For this review, take the finished solid that the model builds, in its own axes (mm). A direction names the side the tool comes from. Coordinates: 2 decimals unless noted, no trailing zeros. Write each loop counter-clockwise with the first axis right and the second up, starting at its lowest first coordinate (ties: lowest second). Pieces come first, ordered by that corner, then holes.
```python
from build123d import *

# Parameters (mm, degrees)
BOSS_EXTRUDE1_DEPTH = 5
SKETCH3_R           = 1.8
SKETCH3_W           = 20
SKETCH3_H           = 3
SKETCH3_W_2         = 25
SKETCH3_W_3         = 3
SKETCH3_H_2         = 30
ARDUINO_DEPTH       = 6
SKETCH6_R           = 1.8
CUT_EXTRUDE4_DEPTH  = 6
SKETCH8_R           = 1.8
CUT_EXTRUDE5_DEPTH  = 10
SKETCH9_R           = 1.8
SKETCH9_R_2         = 2.5
SKETCH9_W           = 3
SKETCH9_H           = 30
L298N_DEPTH         = 10
SKETCH11_W          = 24
SKETCH11_H          = 5
CUT_EXTRUDE7_DEPTH  = 10
SKETCH12_W          = 100
SKETCH12_H          = 20
CUT_EXTRUDE8_DEPTH  = 10


with BuildPart() as part:
    # Sketch1 → Boss-Extrude1 (new body)
    with BuildSketch(Plane(origin=(0, 0, 0), x_dir=(1, 0, 0), z_dir=(0, 1, 0))):
        with BuildLine():
            Line((100, -40), (100, 10))
            Line((100, 10), (30, 170))
            Line((30, 170), (-30, 170))
            Line((-30, 170), (-100, 10))
            Line((-100, 10), (-100, -40))
            ThreePointArc((-100, -40), (-97.071067812, -47.071067812), (-90, -50))
            Line((-90, -50), (-75, -50))
            Line((-75, -50), (-75, -70))
            Line((-75, -70), (-30, -70))
            Line((-30, -70), (-30, -73))
            Line((-30, -73), (30, -73))
            Line((30, -73), (30, -70))
            Line((30, -70), (75, -70))
            Line((75, -70), (75, -50))
            Line((75, -50), (90, -50))
            ThreePointArc((90, -50), (97.071067812, -47.071067812), (100, -40))
        make_face()
    extrude(amount=BOSS_EXTRUDE1_DEPTH)

    # Sketch3 → arduino (cut, through all)
    with BuildSketch(Plane(origin=(0, 5, 0), x_dir=(1, 0, 0), z_dir=(0, 1, 0))):
        with Locations((-76.120983048, 12.737637313)):
            Circle(SKETCH3_R)
        with Locations((-77.220983048, -35.062362687)):
            Circle(SKETCH3_R)
        with Locations((-25.320983048, -2.462362687)):
            Circle(SKETCH3_R)
        with Locations((-25.320983048, -30.362362687)):
            Circle(SKETCH3_R)
        with Locations((-45.320983048, -41.562362687)):
            Rectangle(SKETCH3_W, SKETCH3_H)
        with Locations((-47.820983048, 19.237637313)):
            Rectangle(SKETCH3_W_2, SKETCH3_H)
        with Locations((-18.820983048, -15.362362687)):
            Rectangle(SKETCH3_W_3, SKETCH3_H_2)
    extrude(amount=-ARDUINO_DEPTH, mode=Mode.SUBTRACT)

    # Sketch6 → Cut-Extrude4 (cut, through all)
    with BuildSketch(Plane(origin=(0, 5, 0), x_dir=(1, 0, 0), z_dir=(0, 1, 0))):
        with Locations((20, 120)):
            Circle(SKETCH6_R)
        with Locations((-20, 120)):
            Circle(SKETCH6_R)
    extrude(amount=-CUT_EXTRUDE4_DEPTH, mode=Mode.SUBTRACT)

    # Sketch8 → Cut-Extrude5 (cut)
    with BuildSketch(Plane(origin=(0, 5, 0), x_dir=(1, 0, 0), z_dir=(0, 1, 0))):
        with Locations((8, 10)):
            Circle(SKETCH8_R)
        with Locations((-8, 10)):
            Circle(SKETCH8_R)
        with Locations((-65, -60)):
            Circle(SKETCH8_R)
        with Locations((65, -60)):
            Circle(SKETCH8_R)
        with Locations((8, -52)):
            Circle(SKETCH8_R)
        with Locations((24, -52)):
            Circle(SKETCH8_R)
        with Locations((40, -52)):
            Circle(SKETCH8_R)
        with Locations((-8, -52)):
            Circle(SKETCH8_R)
        with Locations((-40, -52)):
            Circle(SKETCH8_R)
        with Locations((-24, -52)):
            Circle(SKETCH8_R)
    extrude(amount=-CUT_EXTRUDE5_DEPTH, mode=Mode.SUBTRACT)

    # Sketch9 → l298n (cut)
    with BuildSketch(Plane(origin=(0, 5, 0), x_dir=(1, 0, 0), z_dir=(0, 1, 0))):
        with Locations((20, 72)):
            Circle(SKETCH9_R)
        with Locations((-20, 72)):
            Circle(SKETCH9_R)
        with Locations((51, 10)):
            Circle(SKETCH9_R)
        with Locations((87.998174007, 10.367586933)):
            Circle(SKETCH9_R)
        with Locations((88.36576094, -26.630587074)):
            Circle(SKETCH9_R)
        with Locations((51.367586933, -26.998174007)):
            Circle(SKETCH9_R)
        with Locations((-68.125, 50)):
            Circle(SKETCH9_R)
        with Locations((68.125, 50)):
            Circle(SKETCH9_R)
        with Locations((61, 25)):
            Circle(SKETCH9_R_2)
        with Locations((61.367586933, -41.998174007)):
            Circle(SKETCH9_R_2)
        with Locations((0, 27)):
            Circle(SKETCH9_R_2)
        with Locations((29.5, -10)):
            Rectangle(SKETCH9_W, SKETCH9_H)
    extrude(amount=-L298N_DEPTH, mode=Mode.SUBTRACT)

    # Sketch11 → Cut-Extrude7 (cut)
    with BuildSketch(Plane(origin=(0, 5, 0), x_dir=(1, 0, 0), z_dir=(0, 1, 0))):
        with Locations((-58, -67.5)):
            Rectangle(SKETCH11_W, SKETCH11_H)
        with Locations((58, -67.5)):
            Rectangle(SKETCH11_W, SKETCH11_H)
    extrude(amount=-CUT_EXTRUDE7_DEPTH, mode=Mode.SUBTRACT)

    # Sketch12 → Cut-Extrude8 (cut)
    with BuildSketch(Plane(origin=(0, 5, 0), x_dir=(1, 0, 0), z_dir=(0, 1, 0))):
        with Locations((0, 160)):
            Rectangle(SKETCH12_W, SKETCH12_H)
    extrude(amount=-CUT_EXTRUDE8_DEPTH, mode=Mode.SUBTRACT)


solid = part.part
```
Q1. Add section B-B (z = -78). State the section outline as (x, y) points.
Ans:
outline: (-70.25, 0) - (70.25, 0) - (70.25, 5) - (-70.25, 5) - close
Q2. Add section C-C (y = 2.9). Give the number of separate pieces and of enclosed holes in the cut face, then the cut area to 3 significant figures.
Ans:
separate pieces: 1
enclosed holes: 31
area: 33,700 mm2
Q3. Add section D-D (z = -101). State the section outline as (x, y) points, then the cut area to 3 significant figures.
Ans:
outline: (-60.19, 0) - (60.19, 0) - (60.19, 5) - (-60.19, 5) - close
area: 602 mm2
Q4. For probe 1 along Z at (x, y) = (20, 1.5); probe 2 along Z at (x, y) = (8, 3.65); probe 3 along Z at (x, y) = (65, 2.55), list the stretches that pass through material, from the lowest coordinate up.
Ans:
probe 1: z = -150 to -121.8, -118.2 to -73.8, -70.2 to 73
probe 2: z = -150 to -11.8, -8.2 to 50.2, 53.8 to 73
probe 3: z = -90 to 58.2, 61.8 to 65
Q5. Add section A-A (x = -48.5). State the section outline as (y, z) points, then the cut area to 3 significant figures.
Ans:
outline: (0, -127.71) - (5, -127.71) - (5, -20.74) - (0, -20.74) - close; (0, -17.74) - (5, -17.74) - (5, 40.06) - (0, 40.06) - close; (0, 43.06) - (5, 43.06) - (5, 65) - (0, 65) - close
area: 934 mm2
Q6. Clearance check with flat-ended pins moving along their axes: pin 1 Ø4 at (x, z) = (-77.22, 35.06) entering from -Y; pin 2 Ø2 at (y, z) = (3.5, -12.5) entering from -X; pin 3 Ø1.5 at (y, z) = (2.5, 71.5) entering from +X. State where each tip first meets the part, or that it passes through.
Ans:
pin 1: stops at y = 0
pin 2: stops at x = -99.34
pin 3: stops at x = 30
Q7. Draft analysis for pull direction X (two halves, no side actions). For faces 6 (the flat face through (28, 3, 10)), 7 (the flat face through (-17.321, 3, 16)), 8 (the flat face through (-1, 5, -40)), 9 (the flat face through (69.804, 2.465, -79.02)), state which applies: +X half, -X half, draft (parallel to the pull), parting line (faces both ways), or undercut.
Ans:
face 6: undercut
face 7: undercut
face 8: draft
face 9: +X half
Q8. Tool access review of faces 1 (the flat face through (-20.321, 3, 16)), 2 (the flat face through (58, 3, 65)), 3 (the flat face through (-100, 2, 15)), 4 (the flat face through (75, 2, 60)), 5 (the flat face through (-73, 2, 70)): name each direction out of +Z, -Z, +X, -X, +Y, -Y from which nothing blocks a thin tool from reaching the whole face with its end or side.
Ans:
face 1: +Y, -Y
face 2: +Z, +Y, -Y
face 3: +Z, -Z, -X, +Y, -Y
face 4: +Z, +X, +Y, -Y
face 5: +Z, -X, +Y, -Y
